```python
from build123d import *

# Parameters (mm, degrees)
SKETCH_2_R      = 4
EXTRUDE_1_DEPTH = 10
SKETCH_3_W      = 283
SKETCH_3_H      = 10
EXTRUDE_5_DEPTH = 300
SKETCH_6_W      = 283
SKETCH_6_H      = 64.47
SKETCH_6_R      = 4
EXTRUDE_7_DEPTH = 10


with BuildPart() as part:
    # 草图2 → 凸台-拉伸1 (new body)
    with BuildSketch(Plane.XY):
        Polygon((212.655000043, 48), (-50.344999957, 48), (-60.344999957, 48), (-60.344999957, -3.53), (-60.344999957, -6.47), (222.655000043, -6.47), (222.655000043, -3.53), (222.655000043, 48), align=None)
        with Locations((212.655000043, 24)):
            Circle(SKETCH_2_R, mode=Mode.SUBTRACT)
        with Locations((-50.344999957, 24)):
            Circle(SKETCH_2_R, mode=Mode.SUBTRACT)
    extrude(amount=EXTRUDE_1_DEPTH)

    # 草图3 → 凸台-拉伸5 (add)
    with BuildSketch(Plane.XY):
        with Locations((81.155000043, 53)):
            Rectangle(SKETCH_3_W, SKETCH_3_H)
    extrude(amount=EXTRUDE_5_DEPTH)

    # 草图6 → 凸台-拉伸7 (add)
    with BuildSketch(Plane.XY.offset(300)):
        with Locations((81.155000043, 25.765)):
            Rectangle(SKETCH_6_W, SKETCH_6_H)
        with Locations((-50.344999957, 24)):
            Circle(SKETCH_6_R, mode=Mode.SUBTRACT)
        with Locations((212.655000043, 24)):
            Circle(SKETCH_6_R, mode=Mode.SUBTRACT)
    extrude(amount=-EXTRUDE_7_DEPTH)


solid = part.part
```
Part model, mm, in its own coordinate system. A direction names the side the tool comes from. Coordinates: 2 decimals unless noted, no trailing zeros. Loops run counter-clockwise (first coordinate to the right, second up) from the corner with the lowest first, then second, coordinate; pieces in that order, holes last. Notation, with made-up numbers: (55, 56) - (104, 56) arc R38 ccw to (104, 94) - close; hole circle Ø5 at (61.5, 13). An arc over 180 degrees is marked (long way). Write item = value, one per line. Start each with the question number.
Item 1: Cut at C-C, the plane x = 4. Give the cut face in (y, z).
Item 2: 3-axis set-ups, long thin cutter, end or side, ignore diameter. For faces 5 (the flat face through (79, 21, 290)), 6 (the flat face through (79, 26, 300)): which of +Z, -Z, +X, -X, +Y, -Y reach the whole face in a straight line?
Item 3: Cut at A-A, the plane y = 24. Give the cut face in (x, z) (3 decimals), and give its area (3 significant figures).
Item 4: Mould opens along Z. For faces 1 (the flat face through (79, 26, 0)), 2 (the flat face through (79, 48, 148)), 3 (the flat face through (79, -6.47, 5)), 4 (the flat face through (79, 21, 10)) say: released by +Z, released by -Z, zero draft, split by the parting line, or undercut.
Item 5: Flat gauge pins, fed straight in: pin 1 Ø10.5 at (x, y) = (-50.345, 24) entering from +Z; pin 2 Ø5 at (x, z) = (8, 94.5) entering from -Y. Where does each tip first touch, or does it go through?
Item 6: Wall check: L1, parallel to Z at x = 36, y = 9.5; L2, parallel to Y at x = -30.5, z = 41. Give the ranges that are in metal, low to high. Write a range as from..to.
Item 7: Cut at B-B, the plane y = 41. Give the cut face in (x, z) (3 decimals).
Item 8: Cut at D-D, the plane z = 268. Give the cut face in (x, y) (3 decimals), and give its area (3 significant figures).
The answers:
q1.outline = (-6.47, 0) - (58, 0) - (58, 300) - (-6.47, 300) - (-6.47, 290) - (48, 290) - (48, 10) - (-6.47, 10) - close
q2.face_5 = +X, -X, -Y
q2.face_6 = +Z, +X, -X, +Y, -Y
q3.outline = (-60.345, 0) - (-54.345, 0) - (-54.345, 10) - (-60.345, 10) - close; (-60.345, 290) - (-54.345, 290) - (-54.345, 300) - (-60.345, 300) - close; (-46.345, 0) - (208.655, 0) - (208.655, 10) - (-46.345, 10) - close; (-46.345, 290) - (208.655, 290) - (208.655, 300) - (-46.345, 300) - close; (216.655, 0) - (222.655, 0) - (222.655, 10) - (216.655, 10) - close; (216.655, 290) - (222.655, 290) - (222.655, 300) - (216.655, 300) - close
q3.area = 5,340 mm2
q4.face_1 = released by -Z
q4.face_2 = undercut
q4.face_3 = zero draft
q4.face_4 = undercut
q5.pin_1 = 300
q5.pin_2 = 48
q6.L1 = 0..10, 290..300
q6.L2 = 48..58
q7.outline = (-60.345, 0) - (222.655, 0) - (222.655, 10) - (-60.345, 10) - close; (-60.345, 290) - (222.655, 290) - (222.655, 300) - (-60.345, 300) - close
q8.outline = (-60.345, 48) - (222.655, 48) - (222.655, 58) - (-60.345, 58) - close
q8.area = 2,830 mm2
